```python
from build123d import *

# Parameters (mm, degrees)
F1_DEPTH = 18.796


# Not quite as in the source:
# - the program builds the solid bodies; features that only make, move or delete a surface that nothing else refers to are left out


with BuildPart() as f1:
    # F0 (on Front) → F1 (new body)
    with BuildSketch(Plane.XZ):
        Polygon((-34.4498695163, 44.9158253761), (0, 0), (64.659229215, 25.390607867), (39.0626974404, 58.7634295225), align=None)
        Polygon((-103.4818813205, -34.7814559937), (0, 0), (-34.4498695163, 44.9158253761), align=None)
    extrude(amount=F1_DEPTH)


solid = f1.part
```
The model under review builds one solid part; all positions refer to its coordinate system, in mm. Round coordinates to 2 decimals unless told otherwise and drop trailing zeros. Write each loop counter-clockwise with the first axis right and the second up, starting at its lowest first coordinate (ties: lowest second). Pieces come first, ordered by that corner, then holes. Notation, with made-up numbers: (18, 10.5) - (52, 10.5) arc R13 ccw to (52, 20.5) - close; hole circle Ø3 at (69.25, 85). An arc over 180 degrees is marked (long way). Use one line per item in the form item = value.
Q1. Consider section B-B (x = 43). State the section outline as (y, z) points.
Answer key:
outline = (-18.8, 16.89) - (0, 16.89) - (0, 53.63) - (-18.8, 53.63) - close
Q2. Consider section A-A (y = -3.5). State the section outline as (x, z) points.
Answer key:
outline = (-103.48, -34.78) - (0, 0) - (64.66, 25.39) - (39.06, 58.76) - (-34.45, 44.92) - close
Q3. For line 1 (Z direction, x = 43, y = -17); line 2 (Z direction, x = -29.5, y = -1.5); line 3 (X direction, y = -11.5, z = 38), list the stretches that pass through material, from the lowest coordinate up. Write a range as [from, to].
Answer key:
line_1 = [16.89, 53.63]
line_2 = [-9.92, 45.85]
line_3 = [-40.44, 54.99]
Q4. Insertion check: pin 1 Ø8 at (y, z) = (-10, 24) entering from -X; pin 2 Ø2 at (y, z) = (-5, 26) entering from -X; pin 3 Ø1 at (x, y) = (-34.5, -5.5) entering from -Z. Each pin has a flat end and moves straight along its axis. Give the tip position at first contact, or say it passes through.
Answer key:
pin_1 = -56.03
pin_2 = -51.7
pin_3 = -11.76
Q5. Consider section C-C (z = -19.5). State the section outline as (x, y) points, and give its area (3 significant figures).
Answer key:
outline = (-90.25, -18.8) - (-58.02, -18.8) - (-58.02, 0) - (-90.25, 0) - close
area = 606 mm2
